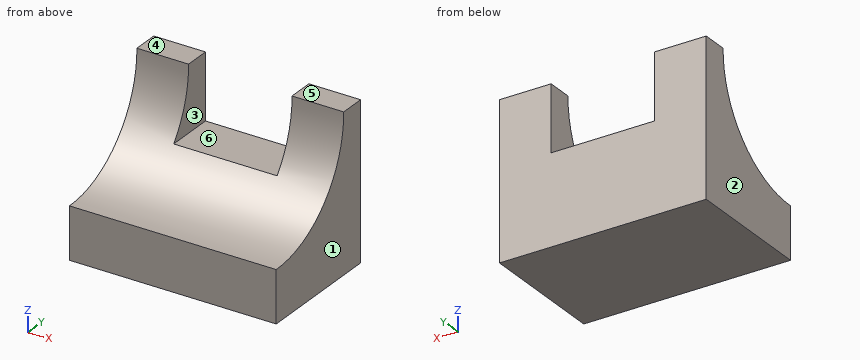
```python
from build123d import *

# Parameters (mm, degrees)
F0_W     = 50.8
F0_H     = 38.1
F1_DEPTH = 31.75
F2_W     = 25.4
F2_H     = 16.111437
F3_DEPTH = 12.7
F5_DEPTH = 50.801


with BuildPart() as f1:
    # F0 (on Front) → F1 (new body)
    with BuildSketch(Plane.XZ):
        with Locations((25.4, 19.05)):
            Rectangle(F0_W, F0_H)
    extrude(amount=F1_DEPTH)

    # F2 (on face) → F3 (cut)
    with BuildSketch(Plane(origin=(0, 0, 0), x_dir=(-1, 0, 0), z_dir=(0, 1, 0))):
        with Locations((-25.4, 30.044282)):
            Rectangle(F2_W, F2_H)
    extrude(amount=-F3_DEPTH, mode=Mode.SUBTRACT)

    # F4 (on face) → F5 (cut, through all)
    with BuildSketch(Plane.YZ.offset(50.8)):
        with BuildLine():
            Line((-31.75, 38.1), (-31.75, 12.7))
            ThreePointArc((-31.75, 12.7), (-13.699472, 20.049472), (-6.35, 38.1))
            Line((-6.35, 38.1), (-31.75, 38.1))
        make_face()
    extrude(amount=-F5_DEPTH, mode=Mode.SUBTRACT)


solid = f1.part
```
The listing builds one solid part. Answer for the finished solid, in the listing's coordinates (mm). Face numbers are marked on the shaded views. A direction names the side the tool comes from. Give positions to 0.01 mm unless a question says otherwise; leave off trailing zeros. Order: outer loops, then holes, each group sorted by start corner. A loop starts at its lowest first (then second) coordinate and runs counter-clockwise, first axis right, second up. Notation, with made-up numbers: (15.25, 29) - (40.25, 29) arc R34 ccw to (40.25, 61) - close; hole circle Ø10 at (14, -24.75). An arc over 180 degrees is marked (long way). Answer in a Markdown table with one row per item. Add a question column.
Q1. The part is cut by section A-A (z = 29). Determine the outline of the cut face in (x, y).
Q2. For a pull along X with two mould halves and no side action, classify the marked faces 1, 2, 3 and 4 as released by +X, released by -X, zero draft, split by the parting line, or undercut.
Q3. The part is cut by section B-B (y = -3.5). Determine the outline of the cut face in (x, z).
Q4. Given P1, Ø5, axis at y = -7, z = 25.5, coming from the -X side; P2, Ø2, axis at x = 29.5, y = -11.5, coming from the +Z side; P3, Ø8, axis at x = 11, z = 21, coming from the -Y side, each flat-ended and moving along its own axis, determine where each tip first touches the part or whether it passes through.
Q5. The part is cut by section D-D (z = 23). Determine the outline of the cut face in (x, y), then the cut area to 3 significant figures.
Q6. Which of the six approach directions +Z, -Z, +X, -X, +Y, -Y give full straight-line access (tool end or side, diameter ignored) to the marked faces 5 and 6?
Q7. The part is cut by section C-C (x = 23). Determine the outline of the cut face in (y, z), then the cut area to 3 significant figures.
Q8. Find the intervals of material crossed by line 1 along X through (y, z) = (-5, 32); line 2 along Z through (x, y) = (24, -8); line 3 along Z through (x, y) = (37.5, -13.5), in increasing order. Write a range as [from, to].
Determined:
| question | item | result |
|---|---|---|
| 1 | outline | (0, -7.94) - (12.7, -7.94) - (12.7, 0) - (0, 0) - close; (38.1, -7.94) - (50.8, -7.94) - (50.8, 0) - (38.1, 0) - close |
| 2 | face 1 | released by +X |
| 2 | face 2 | released by -X |
| 2 | face 3 | undercut |
| 2 | face 4 | zero draft |
| 3 | outline | (0, 0) - (50.8, 0) - (50.8, 38.1) - (38.1, 38.1) - (38.1, 21.99) - (12.7, 21.99) - (12.7, 38.1) - (0, 38.1) - close |
| 4 | P1 | stops at x = 0 |
| 4 | P2 | stops at z = 21.99 |
| 4 | P3 | stops at y = -17.4 |
| 5 | outline | (0, -11.17) - (12.7, -11.17) - (12.7, 0) - (0, 0) - close; (38.1, -11.17) - (50.8, -11.17) - (50.8, 0) - (38.1, 0) - close |
| 5 | area | 284 mm² |
| 6 | face 5 | +Z, +X, -X, +Y, -Y |
| 6 | face 6 | +Z, +Y, -Y |
| 7 | outline | (-31.75, 0) - (0, 0) - (0, 21.99) - (-11.95, 21.99) arc R25.1 cw to (-31.75, 12.7) - close |
| 7 | area | 569 mm² |
| 8 | line 1 | x = [0, 12.7], [38.1, 50.8] |
| 8 | line 2 | z = [0, 21.99] |
| 8 | line 3 | z = [0, 20.25] |
